```python
from build123d import *

# Parameters (mm, degrees)
F0_R          = 31.75
F1_DEPTH      = 5.08
F2_R          = 28.575
F3_DEPTH      = 5.08
F5_DEPTH      = 2.54
F5_DEPTH_BACK = 2.54
F6_R          = 0.381
F8_DEPTH      = 25.4


with BuildPart() as f1:
    # F0 (on Top) → F1 (new body)
    with BuildSketch(Plane.XY):
        Circle(F0_R)
    extrude(amount=F1_DEPTH)

    # F2 (on face) → F3 (cut, through all)
    with BuildSketch(Plane.XY.offset(5.08)):
        Circle(F2_R)
    extrude(amount=-F3_DEPTH, mode=Mode.SUBTRACT)

    # F4 (on Right) → F5 (join, two sides)
    with BuildSketch(Plane.YZ) as f5_sk:
        with BuildLine():
            Line((41.43187, 7.041525), (29.21, 4.699))
            Line((29.21, 4.699), (29.21, 0))
            Line((29.21, 0), (44.45, 0))
            Line((44.45, 0), (44.45, 4.546933))
            ThreePointArc((44.45, 4.546933), (43.528201, 6.504744), (41.43187, 7.041525))
        make_face()
    extrude(amount=F5_DEPTH)
    extrude(f5_sk.sketch, amount=-F5_DEPTH_BACK)

    # F6
    f6_edges = [f1.edges().sort_by_distance(p)[0] for p in [
        (0, 44.45, 0),
    ]]
    fillet(f6_edges, radius=F6_R)

    # F7 (on face) → F8 (cut)
    with BuildSketch(Plane.YZ.offset(2.54)):
        with BuildLine():
            Line((40.400935, 5.550812), (33.02, 4.136133))
            Line((33.02, 4.136133), (33.02, 1.27))
            Line((33.02, 1.27), (41.91, 1.27))
            Line((41.91, 1.27), (41.91, 4.303516))
            ThreePointArc((41.91, 4.303516), (41.449101, 5.282422), (40.400935, 5.550812))
        make_face()
    extrude(amount=-F8_DEPTH, mode=Mode.SUBTRACT)


solid = f1.part
```
Geometry check sheet. Reference: the model listing, model coordinates, mm. A direction names the side the tool comes from. Give positions to 0.01 mm unless a question says otherwise; leave off trailing zeros. Order: outer loops, then holes, each group sorted by start corner. A loop starts at its lowest first (then second) coordinate and runs counter-clockwise, first axis right, second up. Notation, with made-up numbers: (71.25, 34) - (91.25, 34) arc R22 cw to (91.25, 70) - close; hole circle Ø4 at (30, 49.5). An arc over 180 degrees is marked (long way). Answer in a Markdown table with one row per item. Add a question column.
Q1. Cross-section at A-A, the plane z = 2.5. Enter the section's corners in (x, y) (3 decimals), then the cut area to 3 significant figures.
Q2. Gauge pin test, flat ends, axial feed: pin 1 (1.5 mm diameter, centred on x = 0.5, y = 35.5, fed in from +Z); pin 2 (4 mm diameter, centred on x = -25, z = 6, fed in from -Y); pin 3 (4 mm diameter, centred on x = 18, z = 3.5, fed in from -Y). Record the tip position at first contact, or that the pin passes through.
Q3. Cross-section at C-C, the plane y = 0. Enter the section's corners in (x, z) (3 decimals).
Q4. Mould release check, pull along X, two halves, no side actions. Record for faces 1 (the flat face through (-2.54, 38, 1)), 2 (the flat face through (0, 41.91, 3)), 3 (the cylindrical face through (-28.547, 1.256, 2.576)): pulls with the +X half, pulls with the -X half, needs draft (parallel to the pull), parting line crosses it, or undercut.
Q5. Tool access check on faces 4 (the flat face through (0, 36, 6)), 5 (the flat face through (0, 37, 1.27)). Record the directions out of +Z, -Z, +X, -X, +Y, -Y that give a thin tool (end or side, any length) a straight path to the whole face; none if there is none.
Q6. Cross-section at B-B, the plane x = 0. Enter the section's corners in (y, z) (3 decimals).
Q7. Material ranges on probe 1 along X at (y, z) = (32.5, 1); probe 2 along X at (y, z) = (-19, 2.5); probe 3 along Y at (x, z) = (18, 1.75), recorded low to high. Write a range as from..to.
Q8. Cross-section at D-D, the plane x = -16. Enter the section's corners in (y, z), then the cut area to 3 significant figures.
Check values:
| question | item | result |
|---|---|---|
| 1 | outline | (-2.54, 31.648) arc R31.75 ccw (long way) to (2.54, 31.648) - (2.54, 33.02) - (-2.54, 33.02) - close; (-2.54, 41.91) - (2.54, 41.91) - (2.54, 44.45) - (-2.54, 44.45) - close; hole circle Ø57.15 at (0, 0) |
| 1 | area | 621 mm^2 |
| 2 | pin 1 | stops at z = 6.05 |
| 2 | pin 2 | stops at y = -21.65 |
| 2 | pin 3 | stops at y = -27.42 |
| 3 | outline | (-31.75, 0) - (-28.575, 0) - (-28.575, 5.08) - (-31.75, 5.08) - close; (28.575, 0) - (31.75, 0) - (31.75, 5.08) - (28.575, 5.08) - close |
| 4 | face 1 | pulls with the -X half |
| 4 | face 2 | needs draft |
| 4 | face 3 | undercut |
| 5 | face 4 | +Z, +X, -X, -Y |
| 5 | face 5 | +X, -X |
| 6 | outline | (-31.75, 0) - (-28.575, 0) - (-28.575, 5.08) - (-31.75, 5.08) - close; (28.575, 0) - (44.069, 0) arc R0.381 ccw to (44.45, 0.381) - (44.45, 4.547) arc R2.54 ccw to (41.432, 7.042) - (31.198, 5.08) - (28.575, 5.08) - close; hole (33.02, 1.27) - (41.91, 1.27) - (41.91, 4.304) arc R1.27 ccw to (40.401, 5.551) - (33.02, 4.136) - close |
| 7 | probe 1 | x = -2.54..2.54 |
| 7 | probe 2 | x = -25.44..-21.34, 21.34..25.44 |
| 7 | probe 3 | y = -26.15..-22.19, 22.19..26.15 |
| 8 | outline | (-27.42, 0) - (-23.68, 0) - (-23.68, 5.08) - (-27.42, 5.08) - close; (23.68, 0) - (27.42, 0) - (27.42, 5.08) - (23.68, 5.08) - close |
| 8 | area | 38.1 mm^2 |
